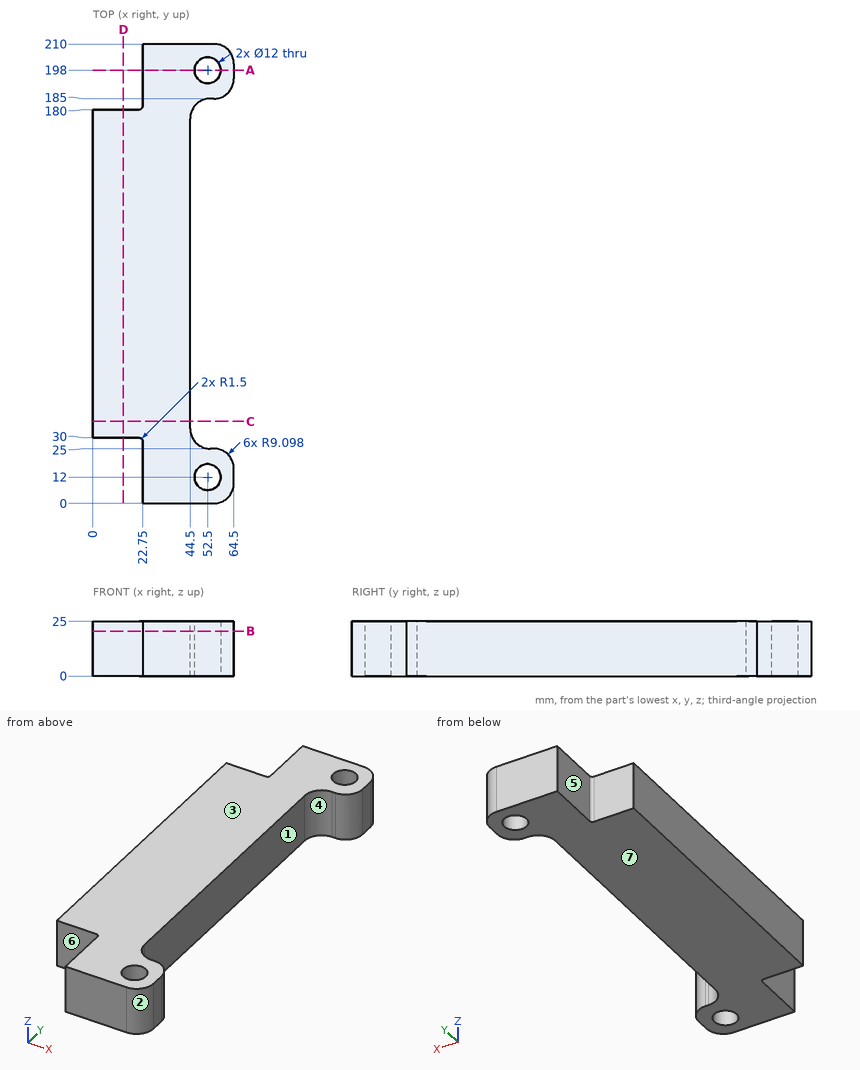
For this review, use the dimensioned drawing (mm, ordinates from the lowest corner) and the shaded views. A direction names the side the tool comes from. Give positions to 0.01 mm unless a question says otherwise; leave off trailing zeros. Order: outer loops, then holes, each group sorted by start corner. A loop starts at its lowest first (then second) coordinate and runs counter-clockwise, first axis right, second up. Notation, with made-up numbers: (-0.75, 42) -> (28.25, 42) arc R15 cw to (28.25, 57) -> close; hole circle Ø11 at (-36.75, 56). An arc over 180 degrees is marked (long way). Write item = value, one per line. Start each with the question number.
(1) Take a section at A-A (y = 198). Write out the cut boundary in (x, z), plus the area to 3 significant figures.
(2) For pin 1 Ø1 at (y, z) = (101, 17.5) entering from +X; pin 2 Ø6 at (y, z) = (76, 7.5) entering from -X; pin 3 Ø7.5 at (y, z) = (9, 18.5) entering from -X; pin 4 Ø6.5 at (x, z) = (13.5, 10) entering from -Y, all flat-tipped, find the tip position at first contact; note any pin that passes through.
(3) Take a section at B-B (z = 20.5). Write out the cut boundary in (x, y).
(4) Take a section at C-C (y = 37.5). Write out the cut boundary in (x, z).
(5) Tool access review of the marked faces 4, 5, 6 and 7: name each direction out of +Z, -Z, +X, -X, +Y, -Y from which nothing blocks a thin tool from reaching the whole face with its end or side.
(6) Take a section at D-D (x = 14). Write out the cut boundary in (y, z).
(7) Draft analysis for pull direction Y (two halves, no side actions). For the marked faces 1, 2 and 3, state which applies: +Y half, -Y half, draft (parallel to the pull), parting line (faces both ways), or undercut.
(8) For L1, parallel to X at y = 197.5, z = 3; L2, parallel to Y at x = 48, z = 18.5 (1 decimal); L3, parallel to Y at x = 49.5, z = 6.75 (1 decimal), list the stretches that pass through material, from the lowest coordinate up. Write a range as from..to.
Returned:
q1.outline = (22.75, 0) -> (46.5, 0) -> (46.5, 25) -> (22.75, 25) -> close; (58.5, 0) -> (64.5, 0) -> (64.5, 25) -> (58.5, 25) -> close
q1.area = 744 mm²
q2.pin_1 = 44.5
q2.pin_2 = 0
q2.pin_3 = 22.75
q2.pin_4 = 30
q3.outline = (0, 30) -> (21.25, 30) arc R1.5 cw to (22.75, 28.5) -> (22.75, 0) -> (55.4, 0) arc R9.1 ccw to (64.5, 9.1) -> (64.5, 15.9) arc R9.1 ccw to (55.4, 25) -> (53.6, 25) arc R9.1 cw to (44.5, 34.1) -> (44.5, 175.9) arc R9.1 cw to (53.6, 185) -> (55.4, 185) arc R9.1 ccw to (64.5, 194.1) -> (64.5, 200.9) arc R9.1 ccw to (55.4, 210) -> (22.75, 210) -> (22.75, 181.5) arc R1.5 cw to (21.25, 180) -> (0, 180) -> close; hole circle Ø12 at (52.5, 12); hole circle Ø12 at (52.5, 198)
q4.outline = (0, 0) -> (44.5, 0) -> (44.5, 25) -> (0, 25) -> close
q5.face_4 = +Z, -Z, +X
q5.face_5 = +Z, -Z, -X, +Y
q5.face_6 = +Z, -Z, -X, -Y
q5.face_7 = -Z, +X, -X, +Y, -Y
q6.outline = (30, 0) -> (180, 0) -> (180, 25) -> (30, 25) -> close
q7.face_1 = undercut
q7.face_2 = -Y half
q7.face_3 = draft
q8.L1 = 22.75..46.52, 58.48..64.5
q8.L2 = 0..8, 16..26.9, 183.1..194, 202..210
q8.L3 = 0..6.8, 17.2..26, 184..192.8, 203.2..210
